Check sheet for the modelled part. Datum: model origin and axes. Units: mm. A direction names the side the tool comes from. Round coordinates to 2 decimals unless told otherwise and drop trailing zeros. Loops run counter-clockwise (first coordinate to the right, second up) from the corner with the lowest first, then second, coordinate; pieces in that order, holes last. Notation, with made-up numbers: M -2,48 L 18,48 A29 ccw 18,72 Z; hole C 81,21.25 d1. An arc over 180 degrees is marked long. Write item = value, one per line. Start each with the question number.
(1) Cross-section at C-C on x = -24.75. Record the boundary of the cut face in (y, z).
(2) Set-up check for faces 1 (the face through (-18, 11.392, 2)), 2 (the face through (-22, 9, 0)), 3 (the face through (-18, 7.392, 2)): record each of +Z, -Z, +X, -X, +Y, -Y from which the full face is reachable in a straight line by a thin tool's end or side.
(3) Scan lines: L1, parallel to X at y = 9.5, z = 2.8; L2, parallel to Y at x = -24.75, z = 0.55; L3, parallel to Y at x = -19, z = 1. Record each from-to range of solid material in increasing order. Write a range as from..to.
(4) Cross-section at D-D on x = -18. Record the boundary of the cut face in (y, z).
(5) Cross-section at B-B on y = 10.5. Record the boundary of the cut face in (x, z), plus the area to 3 significant figures.
(6) Cross-section at A-A on z = 0.9. Record the boundary of the cut face in (x, y) (3 decimals), plus the area to 3 significant figures.
(7) Go/stop test with flat-tipped pins: P1, Ø4, axis at x = -24.24, y = 9.41, coming from the +Z side; P2, Ø0.9, axis at y = 12.5, z = 1.5, coming from the +X side; P3, Ø1, axis at x = -18, y = 6.5, coming from the -Z side. Record where each tip stops, or that it passes through.
(8) Mould release check, pull along Y, two halves, no side actions. Record for faces 4 (the face through (-23.25, 10.175, 1.528)), 5 (the face through (-22, 13.267, 2)), 6 (the face through (-19.192, 6, 2)): pulls with the +Y half, pulls with the -Y half, needs draft (parallel to the pull), parting line crosses it, or undercut.
from build123d import *

# Parameters (mm, degrees)
SKETCH1_R      = 1.25
EXTRUDE1_DEPTH = 3.1


with BuildPart() as part:
    # Sketch1 → Extrude1 (new body)
    with BuildSketch(Plane.XY):
        with BuildLine():
            Line((-19.191802054, 13.266728144), (-19.191802054, 11.391728144))
            Line((-19.191802054, 11.391728144), (-16.091802054, 11.391728144))
            Line((-16.091802054, 11.391728144), (-16.091802054, 7.391728144))
            Line((-16.091802054, 7.391728144), (-19.191802054, 7.391728144))
            Line((-19.191802054, 7.391728144), (-19.191802054, 5.516728144))
            Line((-19.191802054, 5.516728144), (-24.241802054, 5.516728144))
            ThreePointArc((-24.241802054, 5.516728144), (-28.116802054, 9.391728144), (-24.241802054, 13.266728144))
            Line((-24.241802054, 13.266728144), (-19.191802054, 13.266728144))
        make_face()
        with Locations(Location((-24.241802054, 9.414269496, 0), (0, 0, 180))):
            Circle(SKETCH1_R, mode=Mode.SUBTRACT)
    extrude(amount=EXTRUDE1_DEPTH)


solid = part.part
Result:
q1.outline = M 5.55,0 L 8.27,0 L 8.27,3.1 L 5.55,3.1 Z; M 10.56,0 L 13.23,0 L 13.23,3.1 L 10.56,3.1 Z
q2.face_1 = +Z, -Z, +X, +Y
q2.face_2 = -Z, +X, -X, +Y, -Y
q2.face_3 = +Z, -Z, +X, -Y
q3.L1 = -28.12..-25.49, -22.99..-16.09
q3.L2 = 5.55..8.27, 10.56..13.23
q3.L3 = 7.39..11.39
q4.outline = M 7.39,0 L 11.39,0 L 11.39,3.1 L 7.39,3.1 Z
q5.outline = M -27.95,0 L -24.86,0 L -24.86,3.1 L -27.95,3.1 Z; M -23.62,0 L -16.09,0 L -16.09,3.1 L -23.62,3.1 Z
q5.area = 32.9 mm^2
q6.outline = M -24.242,5.517 L -19.192,5.517 L -19.192,7.392 L -16.092,7.392 L -16.092,11.392 L -19.192,11.392 L -19.192,13.267 L -24.242,13.267 A3.875 ccw Z; hole C -24.242,9.414 d2.5
q6.area = 70.2 mm^2
q7.P1 = 3.1
q7.P2 = -19.19
q7.P3 = through
q8.face_4 = undercut
q8.face_5 = pulls with the +Y half
q8.face_6 = needs draft
